from build123d import *

# Parameters (mm, degrees)
F0_W     = 125
F0_H     = 100
F0_R     = 19.05
F1_DEPTH = 89.916


with BuildPart() as f1:
    # F0 (on Front) → F1 (new body)
    with BuildSketch(Plane.XZ):
        Rectangle(F0_W, F0_H)
        Polygon((35.031748, -6.038517), (42.241403, -27.583478), (23.978834, -41.098026), (5.48229, -27.905516), (12.313367, -6.237548), align=None, mode=Mode.SUBTRACT)
        with Locations((-39.0625, 27.042078)):
            Circle(F0_R, mode=Mode.SUBTRACT)
    extrude(amount=F1_DEPTH)


solid = f1.part
Geometry: final body of the model. Coordinates: model frame, mm. A direction names the side the tool comes from. Give positions to 0.01 mm unless a question says otherwise; leave off trailing zeros. Loops run counter-clockwise (first coordinate to the right, second up) from the corner with the lowest first, then second, coordinate; pieces in that order, holes last. Notation, with made-up numbers: (81.25, 38.5) - (87.25, 38.5) arc R22 cw to (87.25, 53.5) - close; hole circle Ø3 at (-29.5, 6.25). An arc over 180 degrees is marked (long way). Answer as CSV lines item,"result". Start each with the question number.
1. Draft query along X for faces 1 (the face through (62.5, -44, -1)), 2 (the face through (38.6, -44.3, -16.7)), 3 (the face through (-1, 0, 1)). Return one class per face: released by +X, released by -X, zero draft, split by the parting line, or undercut.
2. Section A-A, the plane x = 21. Return loops of the section in (y, z).
3. Ray query, L1, parallel to X at y = -44, z = -36; L2, parallel to X at y = -82.5, z = 21; L3, parallel to Z at x = 31, y = -43. Return the intervals inside material, ascending.
4. Reachability of faces 4 (the face through (14.86, -44.329, -34.594)), 5 (the face through (-1, -89.916, 1)) from +Z, -Z, +X, -X, +Y, -Y: full face, straight path, thin tool, end or side. Return the list, or none.
5. Section B-B, the plane z = -22.5. Return loops of the section in (x, y), plus the area to 3 significant figures.
6. Section C-C, the plane y = -41. Return loops of the section in (x, z).
Answers:
1,face 1,"released by +X"
1,face 2,"undercut"
1,face 3,"zero draft"
2,outline,"(-89.92, -50) - (0, -50) - (0, -38.97) - (-89.92, -38.97) - close; (-89.92, -6.16) - (0, -6.16) - (0, 50) - (-89.92, 50) - close"
3,L1,"x = -62.5 to 16.83, 30.87 to 62.5"
3,L2,"x = -62.5 to -57.13, -21 to 62.5"
3,L3,"z = -50 to -35.9, -6.07 to 50"
4,face 4,"+Y, -Y"
4,face 5,"+Z, -Z, +X, -X, -Y"
5,outline,"(-62.5, -89.92) - (7.19, -89.92) - (7.19, 0) - (-62.5, 0) - close; (40.54, -89.92) - (62.5, -89.92) - (62.5, 0) - (40.54, 0) - close"
5,area,"8,240 mm2"
6,outline,"(-62.5, -50) - (62.5, -50) - (62.5, 50) - (-62.5, 50) - close; hole circle Ø38.1 at (-39.06, 27.04); hole (5.48, -27.91) - (23.98, -41.1) - (42.24, -27.58) - (35.03, -6.04) - (12.31, -6.24) - close"
